```python
from build123d import *

# Parameters (mm, degrees)
SKETCH1_W                       = 100
SKETCH1_H                       = 140
BOSS_EXTRUDE1_DEPTH             = 25
SKETCH2_W                       = 100
SKETCH2_H                       = 55
CUT_EXTRUDE1_DEPTH              = 5
CUT_EXTRUDE2_DEPTH              = 5
SKETCH5_R                       = 4
CUT_EXTRUDE3_DEPTH              = 10
M8X1_0_TAPPED_HOLE1_D           = 7
M8X1_0_TAPPED_HOLE1_DEPTH       = 12.896987833
M8X1_0_TAPPED_HOLE1_CSINK_D     = 8.05
M8X1_0_TAPPED_HOLE1_CSINK_ANGLE = 90
M8X1_0_TAPPED_HOLE1_TIP         = 2.103012167
CUT_EXTRUDE4_DEPTH              = 7


with BuildPart() as part:
    # Sketch1 → Boss-Extrude1 (new body)
    with BuildSketch(Plane(origin=(0, 0, 0), x_dir=(1, 0, 0), z_dir=(0, 1, 0))):
        with Locations((-187.409638554, 78.222891566)):
            Rectangle(SKETCH1_W, SKETCH1_H)
    extrude(amount=BOSS_EXTRUDE1_DEPTH)

    # Sketch2 → Cut-Extrude1 (cut)
    with BuildSketch(Plane(origin=(0, 25, 0), x_dir=(1, 0, 0), z_dir=(0, 1, 0))):
        with Locations((-187.409638554, 35.722891566)):
            Rectangle(SKETCH2_W, SKETCH2_H)
    extrude(amount=-CUT_EXTRUDE1_DEPTH, mode=Mode.SUBTRACT)

    # Sketch3 → Cut-Extrude2 (cut)
    with BuildSketch(Plane(origin=(0, 25, 0), x_dir=(1, 0, 0), z_dir=(0, 1, 0))):
        with BuildLine():
            Line((-237.409638554, 148.222891566), (-237.409638554, 63.222891566))
            Line((-237.409638554, 63.222891566), (-232.409638554, 63.222891566))
            Line((-232.409638554, 63.222891566), (-232.409638554, 143.222891566))
            Line((-232.409638554, 143.222891566), (-157.409638554, 143.222891566))
            ThreePointArc((-157.409638554, 143.222891566), (-146.803036836, 138.829493284), (-142.409638554, 128.222891566))
            Line((-142.409638554, 128.222891566), (-142.409638554, 73.222891566))
            ThreePointArc((-142.409638554, 73.222891566), (-149.480706366, 70.293959378), (-152.409638554, 63.222891566))
            Line((-152.409638554, 63.222891566), (-137.409638554, 63.222891566))
            Line((-137.409638554, 63.222891566), (-137.409638554, 148.222891566))
            Line((-137.409638554, 148.222891566), (-237.409638554, 148.222891566))
        make_face()
        with BuildLine():
            ThreePointArc((-192.409638554, 68.222891566), (-193.874104648, 64.68735766), (-197.409638554, 63.222891566))
            Line((-197.409638554, 63.222891566), (-177.409638554, 63.222891566))
            ThreePointArc((-177.409638554, 63.222891566), (-180.94517246, 64.68735766), (-182.409638554, 68.222891566))
            ThreePointArc((-182.409638554, 68.222891566), (-187.409638554, 73.222891566), (-192.409638554, 68.222891566))
        make_face()
    extrude(amount=-CUT_EXTRUDE2_DEPTH, mode=Mode.SUBTRACT)

    # Sketch5 → Cut-Extrude3 (cut)
    with BuildSketch(Plane(origin=(0, 25, 0), x_dir=(1, 0, 0), z_dir=(0, 1, 0))):
        with BuildLine():
            ThreePointArc((-165.409638554, 128.222891566), (-169.409638554, 132.222891566), (-173.409638554, 128.222891566))
            Line((-173.409638554, 128.222891566), (-169.409638554, 128.222891566))
            Line((-169.409638554, 128.222891566), (-165.409638554, 128.222891566))
        make_face()
        with BuildLine():
            Line((-169.409638554, 128.222891566), (-173.409638554, 128.222891566))
            ThreePointArc((-173.409638554, 128.222891566), (-169.409638554, 124.222891566), (-165.409638554, 128.222891566))
            Line((-165.409638554, 128.222891566), (-169.409638554, 128.222891566))
        make_face()
        with Locations(Location((-157.409638554, 128.222891566, 0), (0, 0, 270))):
            Circle(SKETCH5_R)
    extrude(amount=-CUT_EXTRUDE3_DEPTH, mode=Mode.SUBTRACT)

    # M8x1.0 Tapped Hole1
    with Locations(Plane(origin=(-211.409638554, 25, -128.222891566), x_dir=(0, 0, 1), z_dir=(0, 1, 0))):
        with Locations((0, 0), (0, 12)):
            CounterSinkHole(M8X1_0_TAPPED_HOLE1_D / 2, M8X1_0_TAPPED_HOLE1_CSINK_D / 2, depth=M8X1_0_TAPPED_HOLE1_DEPTH, counter_sink_angle=M8X1_0_TAPPED_HOLE1_CSINK_ANGLE)
            with Locations((0, 0, -(M8X1_0_TAPPED_HOLE1_DEPTH + M8X1_0_TAPPED_HOLE1_TIP / 2))):  # 118° drill point
                Cone(0, M8X1_0_TAPPED_HOLE1_D / 2, M8X1_0_TAPPED_HOLE1_TIP, mode=Mode.SUBTRACT)

    # Sketch13 → Cut-Extrude4 (cut)
    with BuildSketch(Plane(origin=(0, 25, 0), x_dir=(1, 0, 0), z_dir=(0, 1, 0))):
        with BuildLine():
            Line((-162.409638554, 85.722891566), (-212.409638554, 85.722891566))
            ThreePointArc((-212.409638554, 85.722891566), (-215.94517246, 87.18735766), (-217.409638554, 90.722891566))
            Line((-217.409638554, 90.722891566), (-217.409638554, 110.722891566))
            ThreePointArc((-217.409638554, 110.722891566), (-215.94517246, 114.258425472), (-212.409638554, 115.722891566))
            Line((-212.409638554, 115.722891566), (-162.409638554, 115.722891566))
            ThreePointArc((-162.409638554, 115.722891566), (-158.874104648, 114.258425472), (-157.409638554, 110.722891566))
            Line((-157.409638554, 110.722891566), (-157.409638554, 90.722891566))
            ThreePointArc((-157.409638554, 90.722891566), (-158.874104648, 87.18735766), (-162.409638554, 85.722891566))
        make_face()
    extrude(amount=-CUT_EXTRUDE4_DEPTH, mode=Mode.SUBTRACT)


solid = part.part
```
Check sheet for the modelled part. Datum: model origin and axes. Units: mm. A direction names the side the tool comes from. Give positions to 0.01 mm unless a question says otherwise; leave off trailing zeros. Order: outer loops, then holes, each group sorted by start corner. A loop starts at its lowest first (then second) coordinate and runs counter-clockwise, first axis right, second up. Notation, with made-up numbers: (-30.5, 57) -> (2.5, 57) arc R12 cw to (2.5, 80) -> close; hole circle Ø2 at (23, 68.5). An arc over 180 degrees is marked (long way). Return JSON: item names as keys, results as strings.
1. Cross-section at A-A, the plane y = 22. Record the cut outline in (x, z).
From the geometry:
{"outline": "(-232.41, -143.22) -> (-157.41, -143.22) arc R15 ccw to (-142.41, -128.22) -> (-142.41, -73.22) arc R10 cw to (-152.41, -63.22) -> (-177.41, -63.22) arc R5 ccw to (-182.41, -68.22) arc R5 cw to (-192.41, -68.22) arc R5 ccw to (-197.41, -63.22) -> (-232.41, -63.22) -> close; hole (-217.41, -110.72) arc R5 ccw to (-212.41, -115.72) -> (-162.41, -115.72) arc R5 ccw to (-157.41, -110.72) -> (-157.41, -90.72) arc R5 ccw to (-162.41, -85.72) -> (-212.41, -85.72) arc R5 ccw to (-217.41, -90.72) -> close; hole circle Ø7 at (-211.41, -128.22); hole circle Ø7 at (-199.41, -128.22); hole circle Ø8 at (-169.41, -128.22); hole circle Ø8 at (-157.41, -128.22)"}
2. Mould release check, pull along Z, two halves, no side actions. Record for faces 4 (the flat face through (-187, 18, -101)), 5 (the flat face through (-232.41, 23, -103)), 6 (the flat face through (-215, 23, -63.223)): +Z half, -Z half, draft (parallel to the pull), parting line (faces both ways), or undercut.
From the geometry:
{"face 4": "undercut", "face 5": "draft", "face 6": "+Z half"}
3. Go/stop test with flat-tipped pins: P1, Ø15, axis at x = -188.5, z = -99.5, coming from the +Y side; P2, Ø1.5, axis at x = -161, y = 22.5, coming from the +Z side; P3, Ø4, axis at y = 23.5, z = -92, coming from the +X side. Record where each tip stops, or that it passes through.
From the geometry:
{"P1": "y = 18", "P2": "z = -63.22", "P3": "x = -142.41"}
4. Cross-section at D-D, the plane z = -118. Record the cut outline in (x, y).
From the geometry:
{"outline": "(-237.41, 0) -> (-137.41, 0) -> (-137.41, 20) -> (-142.41, 20) -> (-142.41, 25) -> (-232.41, 25) -> (-232.41, 20) -> (-237.41, 20) -> close"}
5. Cross-section at C-C, the plane x = -171. Record the cut outline in (y, z).
From the geometry:
{"outline": "(0, -148.22) -> (20, -148.22) -> (20, -143.22) -> (25, -143.22) -> (25, -131.89) -> (15, -131.89) -> (15, -124.55) -> (25, -124.55) -> (25, -115.72) -> (18, -115.72) -> (18, -85.72) -> (25, -85.72) -> (25, -63.22) -> (20, -63.22) -> (20, -8.22) -> (0, -8.22) -> close"}
6. Set-up check for faces 1 (the flat face through (-165, 23, -63.223)), 2 (the flat face through (-187, 22, -85.723)), 3 (the flat face through (-142.41, 23, -101)): record each of +Z, -Z, +X, -X, +Y, -Y from which the full face is reachable in a straight line by a thin tool's end or side.
From the geometry:
{"face 1": "+Z, +X, -X, +Y", "face 2": "+Y", "face 3": "+Z, -Z, +X, +Y"}
7. Cross-section at B-B, the plane z = -88. Record the cut outline in (x, y).
From the geometry:
{"outline": "(-237.41, 0) -> (-137.41, 0) -> (-137.41, 20) -> (-142.41, 20) -> (-142.41, 25) -> (-158.22, 25) -> (-158.22, 18) -> (-216.6, 18) -> (-216.6, 25) -> (-232.41, 25) -> (-232.41, 20) -> (-237.41, 20) -> close"}
8. Material ranges on probe 1 along Z at (x, y) = (-157, 22.5); probe 2 along Y at (x, z) = (-201.5, -50); probe 3 along Z at (x, y) = (-173, 23.25), recorded low to high. Write a range as [from, to].
From the geometry:
{"probe 1": "[-143.22, -132.2], [-124.24, -63.22]", "probe 2": "[0, 20]", "probe 3": "[-143.22, -129.99], [-126.46, -115.72], [-85.72, -63.22]"}
